```python
from build123d import *

# Parameters (mm, degrees)
SKETCH1_W           = 41
SKETCH1_H           = 26
BOSS_EXTRUDE1_DEPTH = 3
SKETCH1_3_W         = 20
SKETCH1_3_H         = 6
SKETCH1_3_W_2       = 7
SKETCH1_3_H_2       = 15
BOSS_EXTRUDE2_DEPTH = 23


with BuildPart() as part:
    # Sketch1 → Boss-Extrude1 (new body)
    with BuildSketch(Plane.XY):
        Rectangle(SKETCH1_W, SKETCH1_H)
    extrude(amount=-BOSS_EXTRUDE1_DEPTH)

    # Sketch1<3> → Boss-Extrude2 (add)
    with BuildSketch(Plane.XY):
        with Locations((-10.5, -16)):
            Rectangle(SKETCH1_3_W, SKETCH1_3_H)
        with Locations((-24, 5.5)):
            Rectangle(SKETCH1_3_W_2, SKETCH1_3_H_2)
        with Locations((24, 5.5)):
            Rectangle(SKETCH1_3_W_2, SKETCH1_3_H_2)
    extrude(amount=-BOSS_EXTRUDE2_DEPTH)


solid = part.part
```
Could you check a few things on this model? Use its own coordinates, in mm. A direction names the side the tool comes from. Coordinates: 2 decimals unless noted, no trailing zeros. Order: outer loops, then holes, each group sorted by start corner. A loop starts at its lowest first (then second) coordinate and runs counter-clockwise, first axis right, second up. Notation, with made-up numbers: M -24.5,-20.75 L -18.5,-20.75 A22 cw -18.5,9.25 Z; hole C 32.25,82 d7. An arc over 180 degrees is marked long. Use a Markdown table: item, result. Add a question column.
Q1. I'm going to push flat-ended pins straight in: pin 1 (8.5 mm diameter, centred on y = -13.5, z = -7.5, fed in from -X); pin 2 (8 mm diameter, centred on x = 15.5, y = -3.5, fed in from -Z); pin 3 (2 mm diameter, centred on x = 23.5, z = -10, fed in from -Y). Where does each tip first touch, or does it pass through?
Q2. I want a section at B-B on y = 4.5. List the corners of the cut face in (x, z) for me.
Q3. If I drill on L1, parallel to X at y = 6, z = -20.25; L2, parallel to Z at x = -12, y = 11; L3, parallel to X at y = -17.5, z = -20.75, over which ranges is the centre line in solid material (lowest first)?
Q4. I want a section at C-C on x = -9.5. List the corners of the cut face in (y, z) for me, then the cut area to 3 significant figures.
Q5. I want a section at A-A on z = -14. List the corners of the cut face in (x, y) for me, then the cut area to 3 significant figures.
Q6. I want a section at D-D on y = -9.5. List the corners of the cut face in (x, z) for me, then the cut area to 3 significant figures.
Q7. Which directions (+Z, -Z, +X, -X, +Y, -Y) give clear straight access to the entire face, cutting with the end or side of a thin tool? Please do faces 1 (the flat face through (20.5, -8, -1)), 2 (the flat face through (20.5, 5, -13)), 3 (the flat face through (0, 0, -3)).
Checked values:
| question | item | result |
|---|---|---|
| 1 | pin 1 | x = -20.5 |
| 1 | pin 2 | z = -3 |
| 1 | pin 3 | y = -2 |
| 2 | outline | M -27.5,-23 L -20.5,-23 L -20.5,-3 L 20.5,-3 L 20.5,-23 L 27.5,-23 L 27.5,0 L -27.5,0 Z |
| 3 | L1 | -27.5 to -20.5, 20.5 to 27.5 |
| 3 | L2 | -3 to 0 |
| 3 | L3 | -20.5 to -0.5 |
| 4 | outline | M -19,-23 L -13,-23 L -13,-3 L 13,-3 L 13,0 L -19,0 Z |
| 4 | area | 216 mm² |
| 5 | outline | M -27.5,-2 L -20.5,-2 L -20.5,13 L -27.5,13 Z; M -20.5,-19 L -0.5,-19 L -0.5,-13 L -20.5,-13 Z; M 20.5,-2 L 27.5,-2 L 27.5,13 L 20.5,13 Z |
| 5 | area | 330 mm² |
| 6 | outline | M -20.5,-3 L 20.5,-3 L 20.5,0 L -20.5,0 Z |
| 6 | area | 123 mm² |
| 7 | face 1 | +Z, -Z, +X, -Y |
| 7 | face 2 | -Z, +Y, -Y |
| 7 | face 3 | -Z, +Y |
